Here's how the part is built. I have some questions about the finished solid (model axes, mm). A direction names the side the tool comes from. Round coordinates to 2 decimals unless told otherwise and drop trailing zeros. Write each loop counter-clockwise with the first axis right and the second up, starting at its lowest first coordinate (ties: lowest second). Pieces come first, ordered by that corner, then holes. Notation, with made-up numbers: (12.25, 41.5) -> (39.25, 41.5) arc R9 cw to (39.25, 58.5) -> close; hole circle Ø5 at (-30.5, -1.75). An arc over 180 degrees is marked (long way). Put each result on its own line as item: value. Start each with the question number.
1) I want a section at C-C, the plane z = -14. Give the number of separate pieces and of enclosed holes in the cut face, then the cut area to 3 significant figures.
2) I want a section at D-D, the plane y = -48.5. List the corners of the cut face in (x, z) for me.
3) I want a section at A-A, the plane z = -59. List the corners of the cut face in (x, y) for me, then the cut area to 3 significant figures.
4) Which directions (+Z, -Z, +X, -X, +Y, -Y) give clear straight access to the entire face, cutting with the end or side of a thin tool? Please do faces 1 (the flat face through (-2, -66.32, -31)), 2 (the cylindrical face through (56.083, 0.237, 18.961)), 3 (the flat face through (31.37, -46.44, -37.57)), 4 (the flat face through (112, -1, -6.174)).
5) If I drill on line 1 along Y through (x, z) = (0, 15); line 2 along Y through (x, z) = (-3, -29.5); line 3 along Y through (x, z) = (-8, 13), over which ranges is the centre line in solid material (lowest first)? Write a range as [from, to].
6) Will these pins go through, and if not, where does the flat tip stop? P1, Ø2, axis at x = 4.5, y = 19, coming from the -Z side; P2, Ø5.5, axis at x = 2, y = -0.5, coming from the +Z side; P3, Ø13.5, axis at y = -5.5, z = -29.5, coming from the +X side.
7) I want a section at B-B, the plane x = 0. List the corners of the cut face in (y, z) for me, then the cut area to 3 significant figures.
8) We'd pull the mould along Y, two halves only. Please class faces 5 (the cylindrical face through (-0.204, -39.355, 18.961)), 6 (the cylindrical face through (-0.229, 33.005, 18.961)): released by +Y, released by -Y, zero draft, split by the parting line, or undercut.
from build123d import *

# Parameters (mm, degrees)
F0_W          = 229.506806
F0_H          = 132.64066
F0_R          = 8.758442
F1_DEPTH      = 12.7
F1_DEPTH_BACK = 76.2
F0_R_2        = 14.221209
F2_DEPTH      = 12.7
F3_DEPTH      = 25.4
F4_DEPTH      = 12.7
F5_W          = 80.183886
F5_H          = 45.04325
F6_DEPTH      = 6.35
F7_R          = 24.948255
F8_DEPTH      = 9.525


with BuildPart() as f1:
    # F0 (on Top) → F1 (new body, two sides)
    with BuildSketch(Plane.XY) as f1_sk:
        Rectangle(F0_W, F0_H)
        with BuildLine():
            ThreePointArc((-66.51097, -11.780334), (-62.431816, 0), (-66.51097, 11.780334))
            Line((-66.51097, 11.780334), (-75.397, 23.073001))
            ThreePointArc((-75.397, 23.073001), (-70.17249, 45.484427), (-47.911137, 51.315352))
            Line((-47.911137, 51.315352), (-14.361814, 41.427133))
            ThreePointArc((-14.361814, 41.427133), (0, 39.354725), (14.361814, 41.427133))
            Line((14.361814, 41.427133), (47.911137, 51.315352))
            ThreePointArc((47.911137, 51.315352), (70.17249, 45.484427), (75.397, 23.073001))
            Line((75.397, 23.073001), (66.51097, 11.780334))
            ThreePointArc((66.51097, 11.780334), (62.431816, 0), (66.51097, -11.780334))
            Line((66.51097, -11.780334), (75.397, -23.073001))
            ThreePointArc((75.397, -23.073001), (70.17249, -45.484427), (47.911137, -51.315352))
            Line((47.911137, -51.315352), (14.361814, -41.427133))
            ThreePointArc((14.361814, -41.427133), (0, -39.354725), (-14.361814, -41.427133))
            Line((-14.361814, -41.427133), (-47.911137, -51.315352))
            ThreePointArc((-47.911137, -51.315352), (-70.17249, -45.484427), (-75.397, -23.073001))
            Line((-75.397, -23.073001), (-66.51097, -11.780334))
        make_face(mode=Mode.SUBTRACT)
        Circle(F0_R)
    extrude(amount=F1_DEPTH)
    extrude(f1_sk.sketch, amount=-F1_DEPTH_BACK)



with BuildPart() as f2:
    # F0 (on Top) → F2 (new body)
    with BuildSketch(Plane.XY):
        with BuildLine():
            ThreePointArc((69.645687, 26.032636), (65.252866, 41.422588), (49.706364, 45.224403))
            Line((49.706364, 45.224403), (16.157041, 35.336183))
            ThreePointArc((16.157041, 35.336183), (0, 33.004725), (-16.157041, 35.336183))
            Line((-16.157041, 35.336183), (-49.706364, 45.224403))
            ThreePointArc((-49.706364, 45.224403), (-65.252866, 41.422588), (-69.645687, 26.032636))
            Line((-69.645687, 26.032636), (-61.520688, 15.707112))
            ThreePointArc((-61.520688, 15.707112), (-56.081816, 0), (-61.520688, -15.707112))
            Line((-61.520688, -15.707112), (-69.645687, -26.032636))
            ThreePointArc((-69.645687, -26.032636), (-65.252866, -41.422588), (-49.706364, -45.224403))
            Line((-49.706364, -45.224403), (-16.157041, -35.336183))
            ThreePointArc((-16.157041, -35.336183), (0, -33.004725), (16.157041, -35.336183))
            Line((16.157041, -35.336183), (49.706364, -45.224403))
            ThreePointArc((49.706364, -45.224403), (65.252866, -41.422588), (69.645687, -26.032636))
            Line((69.645687, -26.032636), (61.520688, -15.707112))
            ThreePointArc((61.520688, -15.707112), (56.081816, 0), (61.520688, 15.707112))
            Line((61.520688, 15.707112), (69.645687, 26.032636))
        make_face()
        Circle(F0_R_2, mode=Mode.SUBTRACT)
    extrude(amount=F2_DEPTH)


with BuildPart() as f1_1:
    add(f1.part)

    add(f2.part)  # F3 merges F2
    # F0 (on Top) → F3 (join)
    with BuildSketch(Plane.XY):
        with BuildLine():
            Line((-75.397, 23.073001), (-66.51097, 11.780334))
            ThreePointArc((-66.51097, 11.780334), (-62.431816, 0), (-66.51097, -11.780334))
            Line((-66.51097, -11.780334), (-75.397, -23.073001))
            ThreePointArc((-75.397, -23.073001), (-70.17249, -45.484427), (-47.911137, -51.315352))
            Line((-47.911137, -51.315352), (-14.361814, -41.427133))
            ThreePointArc((-14.361814, -41.427133), (0, -39.354725), (14.361814, -41.427133))
            Line((14.361814, -41.427133), (47.911137, -51.315352))
            ThreePointArc((47.911137, -51.315352), (70.17249, -45.484427), (75.397, -23.073001))
            Line((75.397, -23.073001), (66.51097, -11.780334))
            ThreePointArc((66.51097, -11.780334), (62.431816, 0), (66.51097, 11.780334))
            Line((66.51097, 11.780334), (75.397, 23.073001))
            ThreePointArc((75.397, 23.073001), (70.17249, 45.484427), (47.911137, 51.315352))
            Line((47.911137, 51.315352), (14.361814, 41.427133))
            ThreePointArc((14.361814, 41.427133), (0, 39.354725), (-14.361814, 41.427133))
            Line((-14.361814, 41.427133), (-47.911137, 51.315352))
            ThreePointArc((-47.911137, 51.315352), (-70.17249, 45.484427), (-75.397, 23.073001))
        make_face()
        with BuildLine():
            Line((16.157041, 35.336183), (49.706364, 45.224403))
            ThreePointArc((49.706364, 45.224403), (65.252866, 41.422588), (69.645687, 26.032636))
            Line((69.645687, 26.032636), (61.520688, 15.707112))
            ThreePointArc((61.520688, 15.707112), (56.081816, 0), (61.520688, -15.707112))
            Line((61.520688, -15.707112), (69.645687, -26.032636))
            ThreePointArc((69.645687, -26.032636), (65.252866, -41.422588), (49.706364, -45.224403))
            Line((49.706364, -45.224403), (16.157041, -35.336183))
            ThreePointArc((16.157041, -35.336183), (0, -33.004725), (-16.157041, -35.336183))
            Line((-16.157041, -35.336183), (-49.706364, -45.224403))
            ThreePointArc((-49.706364, -45.224403), (-65.252866, -41.422588), (-69.645687, -26.032636))
            Line((-69.645687, -26.032636), (-61.520688, -15.707112))
            ThreePointArc((-61.520688, -15.707112), (-56.081816, 0), (-61.520688, 15.707112))
            Line((-61.520688, 15.707112), (-69.645687, 26.032636))
            ThreePointArc((-69.645687, 26.032636), (-65.252866, 41.422588), (-49.706364, 45.224403))
            Line((-49.706364, 45.224403), (-16.157041, 35.336183))
            ThreePointArc((-16.157041, 35.336183), (0, 33.004725), (16.157041, 35.336183))
        make_face(mode=Mode.SUBTRACT)
        Circle(F0_R_2)
        Circle(F0_R, mode=Mode.SUBTRACT)
    extrude(amount=F3_DEPTH)

    # F0 (on Top) → F4 (join)
    with BuildSketch(Plane.XY):
        with BuildLine():
            ThreePointArc((69.645687, 26.032636), (65.252866, 41.422588), (49.706364, 45.224403))
            Line((49.706364, 45.224403), (16.157041, 35.336183))
            ThreePointArc((16.157041, 35.336183), (0, 33.004725), (-16.157041, 35.336183))
            Line((-16.157041, 35.336183), (-49.706364, 45.224403))
            ThreePointArc((-49.706364, 45.224403), (-65.252866, 41.422588), (-69.645687, 26.032636))
            Line((-69.645687, 26.032636), (-61.520688, 15.707112))
            ThreePointArc((-61.520688, 15.707112), (-56.081816, 0), (-61.520688, -15.707112))
            Line((-61.520688, -15.707112), (-69.645687, -26.032636))
            ThreePointArc((-69.645687, -26.032636), (-65.252866, -41.422588), (-49.706364, -45.224403))
            Line((-49.706364, -45.224403), (-16.157041, -35.336183))
            ThreePointArc((-16.157041, -35.336183), (0, -33.004725), (16.157041, -35.336183))
            Line((16.157041, -35.336183), (49.706364, -45.224403))
            ThreePointArc((49.706364, -45.224403), (65.252866, -41.422588), (69.645687, -26.032636))
            Line((69.645687, -26.032636), (61.520688, -15.707112))
            ThreePointArc((61.520688, -15.707112), (56.081816, 0), (61.520688, 15.707112))
            Line((61.520688, 15.707112), (69.645687, 26.032636))
        make_face()
        Circle(F0_R_2, mode=Mode.SUBTRACT)
    extrude(amount=F4_DEPTH)

    # F5 (on face) → F6 (cut)
    with BuildSketch(Plane.YZ.offset(114.753403)):
        with Locations((0, -28.695723)):
            Rectangle(F5_W, F5_H)
    extrude(amount=-F6_DEPTH, mode=Mode.SUBTRACT)

    # F7 (on face) → F8 (cut)
    with BuildSketch(Plane(origin=(-114.753403, 0, 0), x_dir=(0, -1, 0), z_dir=(-1, 0, 0))):
        with Locations((-3.9606, -21.613867)):
            Circle(F7_R)
    extrude(amount=-F8_DEPTH, mode=Mode.SUBTRACT)


solid = f1_1.part
Findings:
1. separate pieces: 2
1. enclosed holes: 1
1. area: 16,500 mm2
2. outline: (-114.75, -76.2) -> (-66.54, -76.2) -> (-66.54, 0) -> (-38.36, 0) -> (-38.36, -76.2) -> (38.36, -76.2) -> (38.36, 0) -> (66.54, 0) -> (66.54, -76.2) -> (114.75, -76.2) -> (114.75, 12.7) -> (66.54, 12.7) -> (66.54, 25.4) -> (38.36, 25.4) -> (38.36, 12.7) -> (-38.36, 12.7) -> (-38.36, 25.4) -> (-66.54, 25.4) -> (-66.54, 12.7) -> (-114.75, 12.7) -> close
3. outline: (-114.75, -66.32) -> (114.75, -66.32) -> (114.75, 66.32) -> (-114.75, 66.32) -> close; circle Ø17.52 at (0, 0); hole (-75.4, -23.07) arc R22.28 ccw to (-47.91, -51.32) -> (-14.36, -41.43) arc R50.8 cw to (14.36, -41.43) -> (47.91, -51.32) arc R22.28 ccw to (75.4, -23.07) -> (66.51, -11.78) arc R19.05 cw to (66.51, 11.78) -> (75.4, 23.07) arc R22.28 ccw to (47.91, 51.32) -> (14.36, 41.43) arc R50.8 cw to (-14.36, 41.43) -> (-47.91, 51.32) arc R22.28 ccw to (-75.4, 23.07) -> (-66.51, 11.78) arc R19.05 cw to (-66.51, -11.78) -> close
3. area: 17,500 mm2
4. face 1: +Z, -Z, +X, -X, -Y
4. face 2: +Z
4. face 3: -Z
4. face 4: +X
5. line 1: y = [-39.35, -33], [-14.22, -8.76], [8.76, 14.22], [33, 39.35]
5. line 2: y = [-66.32, -39.44], [-8.23, 8.23], [39.44, 66.32]
5. line 3: y = [-39.99, -33.57], [-11.76, -3.57], [3.57, 11.76], [33.57, 39.99]
6. P1: stops at z = 0
6. P2: stops at z = 12.7
6. P3: stops at x = 108.4
7. outline: (-66.32, -76.2) -> (-39.35, -76.2) -> (-39.35, 0) -> (-8.76, 0) -> (-8.76, -76.2) -> (8.76, -76.2) -> (8.76, 0) -> (39.35, 0) -> (39.35, -76.2) -> (66.32, -76.2) -> (66.32, 12.7) -> (39.35, 12.7) -> (39.35, 25.4) -> (33, 25.4) -> (33, 12.7) -> (14.22, 12.7) -> (14.22, 25.4) -> (8.76, 25.4) -> (8.76, 12.7) -> (-8.76, 12.7) -> (-8.76, 25.4) -> (-14.22, 25.4) -> (-14.22, 12.7) -> (-33, 12.7) -> (-33, 25.4) -> (-39.35, 25.4) -> (-39.35, 12.7) -> (-66.32, 12.7) -> close
7. area: 7,430 mm2
8. face 5: released by -Y
8. face 6: undercut
